The model under review builds one solid part; all positions refer to its coordinate system, in mm. Face numbers are marked on the shaded views. A direction names the side the tool comes from. Round coordinates to 2 decimals unless told otherwise and drop trailing zeros. Order: outer loops, then holes, each group sorted by start corner. A loop starts at its lowest first (then second) coordinate and runs counter-clockwise, first axis right, second up. Notation, with made-up numbers: M 21,53.25 L 54,53.25 A18 ccw 54,69.25 Z; hole C -26.75,28 d10. An arc over 180 degrees is marked long. Use a Markdown table: item, result. Add a question column.
1. The part is to be moulded in two halves that separate along Y. For the marked faces 4, 5 and 6, say which applies: +Y half, -Y half, draft (parallel to the pull), parting line (faces both ways), or undercut.
2. Consider section B-B on z = 0. State the section outline as (x, y) points, then the cut area to 3 significant figures.
3. Consider section A-A on y = 0. State the section outline as (x, z) points.
4. Insertion check: P1, Ø8, axis at y = 58, z = 10, coming from the +X side; P2, Ø5, axis at y = -2, z = 12.5, coming from the -X side; P3, Ø1.5, axis at x = 16.5, z = -15.5, coming from the +Y side; P4, Ø12, axis at x = 0, y = 58, coming from the -Z side. Each pin has a flat end and moves straight along its axis. Give the tip position at first contact, or say it passes through.
5. Consider section C-C on x = -16. State the section outline as (y, z) points, then the cut area to 3 significant figures.
6. For the marked faces 1, 2 and 3, list the 3-axis set-ups (+Z, -Z, +X, -X, +Y, -Y) from which the entire face can be reached by the end or side of a thin tool; tool diameter is ignored.
7. To check wall thickness, follow probe 1 along Y at (x, z) = (-9, 2); probe 2 along Y at (x, z) = (-5, 0); probe 3 along Y at (x, z) = (16, 8.5). State the ranges of each line that lie inside material, in increasing order.
8. Consider section D-D on x = 12. State the section outline as (y, z) points, then the cut area to 3 significant figures.
from build123d import *

# Parameters (mm, degrees)
SKETCH1_R           = 20
BOSS_EXTRUDE1_DEPTH = 26
BOSS_EXTRUDE2_START = -52
BOSS_EXTRUDE2_DEPTH = 52
CUT_EXTRUDE2_DEPTH  = 26
SKETCH7_R           = 10
CUT_EXTRUDE3_DEPTH  = 52
SKETCH8_R           = 15
CUT_EXTRUDE4_DEPTH  = 52
FILLET1_R           = 0.25


with BuildPart() as part:
    # Sketch1 → Boss-Extrude1 (new, symmetric)
    with BuildSketch(Plane(origin=(0, 0, 0), x_dir=(0, 0, -1), z_dir=(1, 0, 0))):
        with Locations(Location((0, 0, 0), (0, 0, 180))):
            Circle(SKETCH1_R)
    extrude(amount=BOSS_EXTRUDE1_DEPTH, both=True)

    # Sketch4 → Boss-Extrude2 (add)
    with BuildSketch(Plane.ZY.offset(26).offset(BOSS_EXTRUDE2_START)):
        with BuildLine():
            Line((-9.839336332, 20.254001388), (-9.839336332, 78))
            Line((-9.839336332, 78), (9.927883161, 78))
            Line((9.927883161, 78), (9.927883161, 20.254001388))
            ThreePointArc((9.927883161, 20.254001388), (10.473458868, 17.8880874), (12, 16))
            ThreePointArc((12, 16), (0, 20), (-12, 16))
            ThreePointArc((-12, 16), (-10.424631432, 17.875564978), (-9.839336332, 20.254001388))
        make_face()
    extrude(amount=BOSS_EXTRUDE2_DEPTH)

    # Sketch3 → Cut-Extrude2 (cut, symmetric)
    with BuildSketch(Plane.XY):
        with BuildLine():
            Line((-26, 20), (-19.773297574, 61.002782551))
            ThreePointArc((-19.773297574, 61.002782551), (-13.037337707, 73.16666824), (0, 78))
            Line((0, 78), (-26, 78))
            Line((-26, 78), (-26, 20))
        make_face()
    cut_extrude2 = extrude(amount=CUT_EXTRUDE2_DEPTH, both=True, mode=Mode.SUBTRACT)

    # Mirror1: Cut-Extrude2 across plane
    add(cut_extrude2.mirror(Plane(origin=(0, 0, 0), x_dir=(0, 0, 1), z_dir=(1, 0, 0))), mode=Mode.SUBTRACT)

    # Sketch7 → Cut-Extrude3 (cut)
    with BuildSketch(Plane.XY.offset(9.927883161)):
        with Locations((0, 58)):
            Circle(SKETCH7_R)
    extrude(amount=-CUT_EXTRUDE3_DEPTH, mode=Mode.SUBTRACT)

    # Sketch8 → Cut-Extrude4 (cut)
    with BuildSketch(Plane(origin=(26, 0, 0), x_dir=(0, 0, -1), z_dir=(1, 0, 0))):
        Circle(SKETCH8_R)
    extrude(amount=-CUT_EXTRUDE4_DEPTH, mode=Mode.SUBTRACT)

    # Fillet1
    fillet1_edges = [part.edges().sort_by_distance(p)[0] for p in [
        (-10, 58, -9.839336332),
        (-10, 58, 9.927883161),
        (-26, 0, 15),
        (26, 0, 15),
    ]]
    fillet(fillet1_edges, radius=FILLET1_R)


solid = part.part
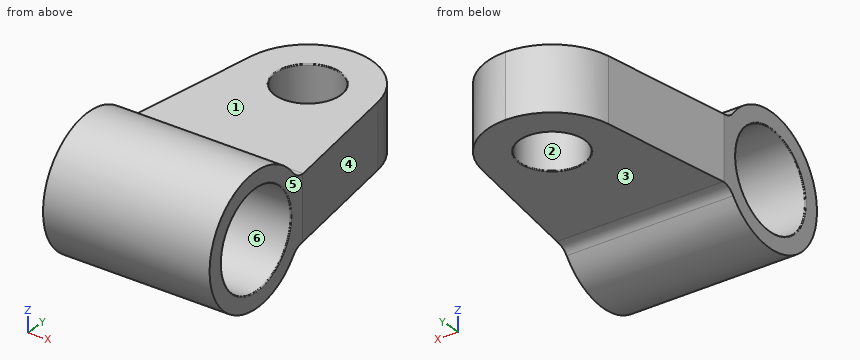
Answer block:
| question | item | result |
|---|---|---|
| 1 | face 4 | +Y half |
| 1 | face 5 | draft |
| 1 | face 6 | undercut |
| 2 | outline | M -26,-20 L 26,-20 L 26,-15.25 A0.25 ccw 25.75,-15 L -25.75,-15 A0.25 ccw -26,-15.25 Z; M -26,15.25 A0.25 ccw -25.75,15 L 25.75,15 A0.25 ccw 26,15.25 L 26,20 L 19.77,61 A20 ccw -19.77,61 L -26,20 Z; hole C 0,58 d20 |
| 2 | area | 2,590 mm^2 |
| 3 | outline | M -26,-20 L 26,-20 L 26,-15.25 A0.25 ccw 25.75,-15 L -25.75,-15 A0.25 ccw -26,-15.25 Z; M -26,15.25 A0.25 ccw -25.75,15 L 25.75,15 A0.25 ccw 26,15.25 L 26,20 L -26,20 Z |
| 4 | P1 | x = 20.84 |
| 4 | P2 | x = -25.98 |
| 4 | P3 | y = 13.51 |
| 4 | P4 | through |
| 5 | outline | M 16,-12 A5.4 cw 20.25,-9.84 L 70,-9.84 L 70,9.93 L 20.25,9.93 A5.4 cw 16,12 A20 ccw long Z; hole C 0,0 d30 |
| 5 | area | 1,560 mm^2 |
| 6 | face 1 | +Z, +X, -X, +Y |
| 6 | face 2 | +Z, -Z |
| 6 | face 3 | -Z, +X, -X, +Y |
| 7 | probe 1 | -19.9 to -14.87, 14.87 to 53.64, 62.36 to 75.86 |
| 7 | probe 2 | -20 to -15, 15 to 49.34, 66.66 to 77.36 |
| 7 | probe 3 | -18.1 to -12.36, 12.36 to 70 |
| 8 | outline | M 16,-12 A5.4 cw 20.25,-9.84 L 74,-9.84 L 74,9.93 L 20.25,9.93 A5.4 cw 16,12 A20 ccw long Z; hole C 0,0 d30 |
| 8 | area | 1,640 mm^2 |
